Here's how the part is built. I have some questions about the finished solid (model axes, mm). A direction names the side the tool comes from. Round coordinates to 2 decimals unless told otherwise and drop trailing zeros. Loops run counter-clockwise (first coordinate to the right, second up) from the corner with the lowest first, then second, coordinate; pieces in that order, holes last. Notation, with made-up numbers: M 53.5,34.5 L 77.5,34.5 A15 cw 77.5,48.5 Z; hole C 69,-13 d1. An arc over 180 degrees is marked long. Use a Markdown table: item, result.
```python
from build123d import *

# Parameters (mm, degrees)
F0_W     = 63.5
F0_H     = 17.78
F1_DEPTH = 8.89
F2_R     = 3.937
F3_DEPTH = 6.35
F4_R     = 3.81


with BuildPart() as f1:
    # F0 (on Top) → F1 (new body)
    with BuildSketch(Plane.XY):
        with Locations((31.75, 8.89)):
            Rectangle(F0_W, F0_H)
    extrude(amount=F1_DEPTH)

    # F2 (on face) → F3 (cut)
    with BuildSketch(Plane.XY.offset(8.89)):
        with Locations((8.89, 8.89)):
            Circle(F2_R)
        with Locations((54.61, 8.89)):
            Circle(F2_R)
    extrude(amount=-F3_DEPTH, mode=Mode.SUBTRACT)

    # F4
    f4_edges = [f1.edges().sort_by_distance(p)[0] for p in [
        (31.75, 0, 8.89),
        (0, 8.89, 8.89),
        (31.75, 17.78, 8.89),
        (63.5, 8.89, 8.89),
    ]]
    fillet(f4_edges, radius=F4_R)


solid = f1.part
```
Q1. For faces 5 (the flat face through (0, 9, 3)), 6 (the cylindrical face through (58.365, 10.073, 5.759)), which set-ups out of +Z, -Z, +X, -X, +Y, -Y let a thin tool reach every point of the face, with its end or its side?
Return value:
| item | result |
|---|---|
| face 5 | +Z, -Z, -X, +Y, -Y |
| face 6 | +Z |
Q2. Imagine slicing it at D-D, the plane x = 7.5. Please give me the cut outline in (y, z), then the cut area to 3 significant figures.
Return value:
| item | result |
|---|---|
| outline | M 0,0 L 17.78,0 L 17.78,5.08 A3.81 ccw 13.97,8.89 L 12.57,8.89 L 12.57,2.54 L 5.21,2.54 L 5.21,8.89 L 3.81,8.89 A3.81 ccw 0,5.08 Z |
| area | 105 mm^2 |
Q3. Imagine slicing it at B-B, the plane x = 54.61. Please give me the cut outline in (y, z), then the cut area to 3 significant figures.
Return value:
| item | result |
|---|---|
| outline | M 0,0 L 17.78,0 L 17.78,5.08 A3.81 ccw 13.97,8.89 L 12.83,8.89 L 12.83,2.54 L 4.95,2.54 L 4.95,8.89 L 3.81,8.89 A3.81 ccw 0,5.08 Z |
| area | 102 mm^2 |
Q4. Will these pins go through, and if not, where does the flat tip stop? P1, Ø4, axis at x = 53.5, y = 8.5, coming from the +Z side; P2, Ø1, axis at x = 56.5, z = 8, coming from the -Y side.
Return value:
| item | result |
|---|---|
| P1 | stops at z = 2.54 |
| P2 | stops at y = 0.87 |
Q5. Imagine slicing it at A-A, the plane z = 3.75. Please give me the cut outline in (x, y), then the cut area to 3 significant figures.
Return value:
| item | result |
|---|---|
| outline | M 0,0 L 63.5,0 L 63.5,17.78 L 0,17.78 Z; hole C 8.89,8.89 d7.87; hole C 54.61,8.89 d7.87 |
| area | 1,030 mm^2 |
Q6. I need wall thicknesses on line 1 (Y direction, x = 54.61, z = 4.75); line 2 (X direction, y = 12.5, z = 8.5); line 3 (X direction, y = 7.25, z = 7). Which ranges of each line are inside material? Lowest first, please. Write a range as from..to.
Return value:
| item | result |
|---|---|
| line 1 | y = 0..4.95, 12.83..17.78 |
| line 2 | x = 2.13..7.32, 10.46..53.04, 56.18..61.37 |
| line 3 | x = 0.52..5.31, 12.47..51.03, 58.19..62.98 |
Q7. Imagine slicing it at C-C, the plane y = 8.89. Please give me the cut outline in (x, z), then the cut area to 3 significant figures.
Return value:
| item | result |
|---|---|
| outline | M 0,0 L 63.5,0 L 63.5,5.08 A3.81 ccw 59.69,8.89 L 58.55,8.89 L 58.55,2.54 L 50.67,2.54 L 50.67,8.89 L 12.83,8.89 L 12.83,2.54 L 4.95,2.54 L 4.95,8.89 L 3.81,8.89 A3.81 ccw 0,5.08 Z |
| area | 458 mm^2 |
Q8. We'd pull the mould along X, two halves only. Please class faces 1 (the flat face through (31, 0, 3)), 2 (the flat face through (55, 9, 2.54)), 3 (the cylindrical face through (1.086, 9.014, 7.744)), 4 (the cylindrical face through (62.354, 9.014, 7.804)): pulls with the +X half, pulls with the -X half, needs draft (parallel to the pull), parting line crosses it, or undercut.
Return value:
| item | result |
|---|---|
| face 1 | needs draft |
| face 2 | undercut |
| face 3 | pulls with the -X half |
| face 4 | pulls with the +X half |
